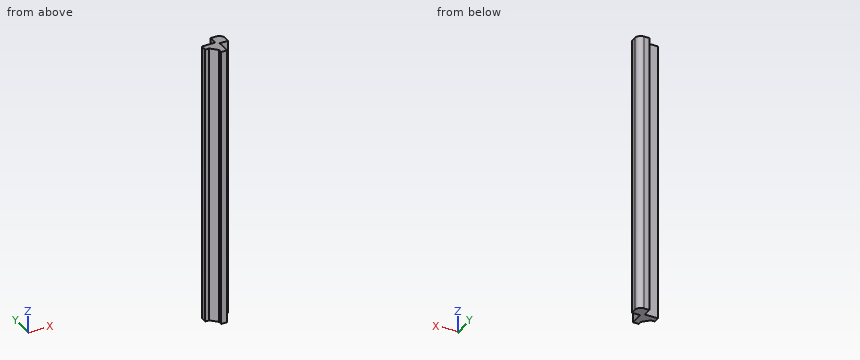
```python
from build123d import *

# Parameters (mm, degrees)
SKETCH7_W           = 4.7625
SKETCH7_H           = 2.12122512
BOSS_EXTRUDE2_DEPTH = 50.27295
SKETCH8_W           = 2.12122512
SKETCH8_H           = 4.7625
BOSS_EXTRUDE3_DEPTH = 50.27295
BOSS_EXTRUDE4_DEPTH = 50.27295


with BuildPart() as part:
    # Sketch7 → Boss-Extrude2 (new, symmetric)
    with BuildSketch(Plane.XY):
        with Locations((-4.92125, -2.560612608)):
            Rectangle(SKETCH7_W, SKETCH7_H)
    extrude(amount=BOSS_EXTRUDE2_DEPTH, both=True)

    # Sketch8 → Boss-Extrude3 (add, symmetric)
    with BuildSketch(Plane.XY):
        with Locations((-2.560612608, -4.92125)):
            Rectangle(SKETCH8_W, SKETCH8_H)
    extrude(amount=BOSS_EXTRUDE3_DEPTH, both=True)

    # Sketch11 → Boss-Extrude4 (add, symmetric)
    with BuildSketch(Plane.XY):
        with BuildLine():
            Line((-2.54, 1.500000048), (-2.54, -1.500000048))
            Line((-2.54, -1.500000048), (-7.3025, -1.500000048))
            Line((-7.3025, -1.500000048), (-7.3025, -3.621225168))
            Line((-7.3025, -3.621225168), (-5.866289198, -3.621225168))
            Line((-5.866289198, -3.621225168), (-3.621225168, -5.866289198))
            Line((-3.621225168, -5.866289198), (-3.621225168, -7.3025))
            Line((-3.621225168, -7.3025), (-1.500000048, -7.3025))
            Line((-1.500000048, -7.3025), (-1.500000048, -2.54))
            Line((-1.500000048, -2.54), (1.500000048, -2.54))
            Line((1.500000048, -2.54), (1.500000048, -0.519999976))
            ThreePointArc((1.500000048, -0.519999976), (0.908355739, 0.908355739), (-0.519999976, 1.500000048))
            Line((-0.519999976, 1.500000048), (-2.54, 1.500000048))
        make_face()
    extrude(amount=BOSS_EXTRUDE4_DEPTH, both=True)


solid = part.part
```
The listing builds one solid part. Answer for the finished solid, in the listing's coordinates (mm). Coordinates: 2 decimals unless noted, no trailing zeros. Write each loop counter-clockwise with the first axis right and the second up, starting at its lowest first coordinate (ties: lowest second). Pieces come first, ordered by that corner, then holes. Notation, with made-up numbers: M 35,42 L 91,42 A15 cw 91,64 Z; hole C 71,-11.5 d4. An arc over 180 degrees is marked long. Use a Markdown table: item, result. Add a question column.
1. Section C-C (y = -4.75) is taken. Give the vertices of the cut face in (x, z).
2. Section A-A (z = 23) is taken. Give the vertices of the cut face in (x, y).
3. Section B-B (x = -4.5) is taken. Give the vertices of the cut face in (y, z).
4. Straight lines are drawn through the part: line 1 along X through (y, z) = (-6.5, -9.5); line 2 along Y through (x, z) = (-3, 40.5). For each, find the intervals that lie inside material, in ascending order. Write a range as [from, to].
5. Given P1, Ø1.1, axis at x = -6.5, z = 13, coming from the -Y side; P2, Ø2.5, axis at y = -4.5, z = 10, coming from the +X side; P3, Ø3, axis at x = -6, z = 14.5, coming from the +Y side, each flat-ended and moving along its own axis, determine where each tip first touches the part or whether it passes through.
Data:
| question | item | result |
|---|---|---|
| 1 | outline | M -4.74,-50.27 L -1.5,-50.27 L -1.5,50.27 L -4.74,50.27 Z |
| 2 | outline | M -7.3,-3.62 L -5.87,-3.62 L -3.62,-5.87 L -3.62,-7.3 L -1.5,-7.3 L -1.5,-2.54 L 1.5,-2.54 L 1.5,-0.52 A2.02 ccw -0.52,1.5 L -2.54,1.5 L -2.54,-1.5 L -7.3,-1.5 Z |
| 3 | outline | M -4.99,-50.27 L -1.5,-50.27 L -1.5,50.27 L -4.99,50.27 Z |
| 4 | line 1 | x = [-3.62, -1.5] |
| 4 | line 2 | y = [-7.3, -1.5] |
| 5 | P1 | stops at y = -3.62 |
| 5 | P2 | stops at x = -1.5 |
| 5 | P3 | stops at y = -1.5 |
